```python
from build123d import *

# Parameters (mm, degrees)
SKETCH1_W           = 56
SKETCH1_H           = 37.25
BOSS_EXTRUDE1_DEPTH = 2
SKETCH2_W           = 56
SKETCH2_H           = 37.25
SKETCH2_W_2         = 52
SKETCH2_H_2         = 33.25
BOSS_EXTRUDE2_DEPTH = 8.5
SKETCH5_W           = 54
SKETCH5_H           = 35.25
SKETCH5_W_2         = 52
SKETCH5_H_2         = 33.25
CUT_EXTRUDE1_DEPTH  = 1
FILLET1_R           = 1
SKETCH7_W           = 30
SKETCH7_H           = 14
CUT_EXTRUDE3_DEPTH  = 10
SKETCH8_R           = 1.75
CUT_EXTRUDE4_DEPTH  = 10
SKETCH9_W           = 7
SKETCH9_H           = 6
CUT_EXTRUDE5_DEPTH  = 3
SKETCH10_W          = 10
SKETCH10_H          = 2.5
CUT_EXTRUDE6_DEPTH  = 3
FILLET2_R           = 0.5
FILLET3_R           = 1
FILLET5_R           = 0.2
CUT_EXTRUDE8_DEPTH  = 0.7
CUT_EXTRUDE10_DEPTH = 5
FILLET6_R           = 0.2


with BuildPart() as part:
    # Sketch1 → Boss-Extrude1 (new body)
    with BuildSketch(Plane(origin=(0, 0, 0), x_dir=(1, 0, 0), z_dir=(0, 1, 0))):
        with Locations((28, 18.625)):
            Rectangle(SKETCH1_W, SKETCH1_H)
    extrude(amount=BOSS_EXTRUDE1_DEPTH)

    # Sketch2 → Boss-Extrude2 (add)
    with BuildSketch(Plane(origin=(0, 2, 0), x_dir=(1, 0, 0), z_dir=(0, 1, 0))):
        with Locations((28, 18.625)):
            Rectangle(SKETCH2_W, SKETCH2_H)
        with Locations((28, 18.625)):
            Rectangle(SKETCH2_W_2, SKETCH2_H_2, mode=Mode.SUBTRACT)
    extrude(amount=BOSS_EXTRUDE2_DEPTH)

    # Sketch5 → Cut-Extrude1 (cut)
    with BuildSketch(Plane(origin=(0, 10.5, 0), x_dir=(1, 0, 0), z_dir=(0, 1, 0))):
        with Locations((28, 18.625)):
            Rectangle(SKETCH5_W, SKETCH5_H)
        with Locations((28, 18.625)):
            Rectangle(SKETCH5_W_2, SKETCH5_H_2, mode=Mode.SUBTRACT)
        with Locations((28, 18.625)):
            Rectangle(SKETCH5_W_2, SKETCH5_H_2)
    extrude(amount=-CUT_EXTRUDE1_DEPTH, mode=Mode.SUBTRACT)

    # Fillet1
    fillet1_edges = [part.edges().sort_by_distance(p)[0] for p in [
        (0, 5.25, -37.25),
        (56, 5.25, -37.25),
        (56, 5.25, 0),
        (0, 5.25, 0),
    ]]
    fillet(fillet1_edges, radius=FILLET1_R)

    # Sketch7 → Cut-Extrude3 (cut)
    with BuildSketch(Plane(origin=(0, 2, 0), x_dir=(1, 0, 0), z_dir=(0, 1, 0))):
        with Locations((31, 13)):
            Rectangle(SKETCH7_W, SKETCH7_H)
    extrude(amount=-CUT_EXTRUDE3_DEPTH, mode=Mode.SUBTRACT)

    # Sketch8 → Cut-Extrude4 (cut)
    with BuildSketch(Plane.XZ):
        with Locations((29.24999924, -23.74999914)):
            Circle(SKETCH8_R)
        with Locations((37.25000102, -23.74999914)):
            Circle(SKETCH8_R)
    extrude(amount=-CUT_EXTRUDE4_DEPTH, mode=Mode.SUBTRACT)

    # Sketch9 → Cut-Extrude5 (cut)
    with BuildSketch(Plane(origin=(0, 0, -37.25), x_dir=(-1, 0, 0), z_dir=(0, 0, -1))):
        with Locations((-47.5, 7.5)):
            Rectangle(SKETCH9_W, SKETCH9_H)
    extrude(amount=-CUT_EXTRUDE5_DEPTH, mode=Mode.SUBTRACT)

    # Sketch10 → Cut-Extrude6 (cut)
    with BuildSketch(Plane(origin=(0, 0, -37.25), x_dir=(-1, 0, 0), z_dir=(0, 0, -1))):
        with Locations((-39, 9.25)):
            Rectangle(SKETCH10_W, SKETCH10_H)
    extrude(amount=-CUT_EXTRUDE6_DEPTH, mode=Mode.SUBTRACT)

    # Fillet2
    fillet2_edges = [part.edges().sort_by_distance(p)[0] for p in [
        (16, 1, -6),
        (16, 1, -20),
        (46, 1, -20),
        (46, 1, -6),
    ]]
    fillet(fillet2_edges, radius=FILLET2_R)

    # Fillet3
    fillet3_edges = [part.edges().sort_by_distance(p)[0] for p in [
        (28, 0, -37.25),
        (0, 0, -18.625),
        (56, 0, -18.625),
        (28, 0, 0),
        (0.292893219, 0, -0.292893219),
        (0.292893219, 0, -36.957106781),
        (55.707106781, 0, -0.292893219),
        (55.707106781, 0, -36.957106781),
    ]]
    fillet(fillet3_edges, radius=FILLET3_R)

    # Fillet5
    fillet5_edges = [part.edges().sort_by_distance(p)[0] for p in [
        (51, 4.5, -36.25),
        (44, 4.5, -36.25),
        (44, 8, -36.25),
        (34, 8, -36.25),
    ]]
    fillet(fillet5_edges, radius=FILLET5_R)

    # Sketch12 → Cut-Extrude8 (cut)
    with BuildSketch(Plane(origin=(0, 9.5, 0), x_dir=(1, 0, 0), z_dir=(0, 1, 0))):
        Polygon((34, 35.25), (34, 36.25), (1, 36.25), (1, 1), (55, 1), (55, 36.25), (51, 36.25), (51, 35.25), (54, 35.25), (54, 2), (2, 2), (2, 35.25), align=None)
    extrude(amount=-CUT_EXTRUDE8_DEPTH, mode=Mode.SUBTRACT)

    # Sketch13 → Cut-Extrude10 (cut)
    with BuildSketch(Plane.ZY):
        Polygon((-18.625, 8.5), (-19.625, 8.5), (-19.625, 10.5), (-17.625, 10.5), (-17.625, 8.5), align=None)
    extrude(amount=-CUT_EXTRUDE10_DEPTH, mode=Mode.SUBTRACT)

    # Fillet6
    fillet6_edges = [part.edges().sort_by_distance(p)[0] for p in [
        (1, 8.5, -17.625),
        (1, 8.5, -19.625),
    ]]
    fillet(fillet6_edges, radius=FILLET6_R)


solid = part.part
```
Can you work these out from the model? Positions are in its coordinate system, mm. A direction names the side the tool comes from. Round coordinates to 2 decimals unless told otherwise and drop trailing zeros. Loops run counter-clockwise (first coordinate to the right, second up) from the corner with the lowest first, then second, coordinate; pieces in that order, holes last. Notation, with made-up numbers: M 49,70.5 L 107,70.5 A19 ccw 107,74.5 Z; hole C -34,13.5 d4. An arc over 180 degrees is marked long. Answer in a Markdown table with one row per item.
1. On a 3-axis mill with a long thin cutter (end or side, diameter ignored), from which of +Z, -Z, +X, -X, +Y, -Y can I reach the whole of each face in a straight line? I mean faces 5 (the face through (28, 5, -2)), 6 (the face through (0.5, 9.6, -17.625)), 7 (the face through (39, 8, -36)), 8 (the face through (46, 1, -13)). Say none if no direction works.
Established:
| item | result |
|---|---|
| face 5 | +Y |
| face 6 | -X, +Y |
| face 7 | -Z, +Y |
| face 8 | +Y, -Y |
2. If we section it at D-D, the plane z = -23.75: Please give me the cut outline in (x, y).
Established:
| item | result |
|---|---|
| outline | M 0,1 A1 ccw 1,0 L 27.5,0 L 27.5,2 L 2,2 L 2,8.8 L 1,8.8 L 1,10.5 L 0,10.5 Z; M 31,0 L 35.5,0 L 35.5,2 L 31,2 Z; M 39,0 L 55,0 A1 ccw 56,1 L 56,10.5 L 55,10.5 L 55,8.8 L 54,8.8 L 54,2 L 39,2 Z |
3. Please list where these lines run through material, in increasing order: line 1 (Z direction, x = 29.25, y = 1.3); line 2 (X direction, y = 10.25, z = -20.5); line 3 (Z direction, x = 6.5, y = 7.5). Write a range as from..to.
Established:
| item | result |
|---|---|
| line 1 | -37.25..-25.5, -22..-20, -6..0 |
| line 2 | 0..1, 55..56 |
| line 3 | -37.25..-35.25, -2..0 |
4. If we section it at B-B, the plane x = 29.25: Please give me the cut outline in (y, z).
Established:
| item | result |
|---|---|
| outline | M 0,-36.25 A1 ccw 1,-37.25 L 10.5,-37.25 L 10.5,-36.25 L 8.8,-36.25 L 8.8,-35.25 L 2,-35.25 L 2,-25.5 L 0,-25.5 Z; M 0,-22 L 2,-22 L 2,-20 L 0,-20 Z; M 0,-6 L 2,-6 L 2,-2 L 8.8,-2 L 8.8,-1 L 10.5,-1 L 10.5,0 L 1,0 A1 ccw 0,-1 Z |
5. I'm going to push flat-ended pins straight in: pin 1 Ø0.5 at (x, y) = (0.5, 9.5) entering from -Z; pin 2 Ø0.6 at (x, z) = (38.5, -36.5) entering from +Y; pin 3 Ø3 at (x, z) = (47, -26) entering from +Y; pin 4 Ø2 at (x, z) = (37.25, -23.75) entering from -Y. Where does each tip first touch, or does it pass through?
Established:
| item | result |
|---|---|
| pin 1 | z = -37.22 |
| pin 2 | y = 8 |
| pin 3 | y = 2 |
| pin 4 | through |
6. Thinking about a two-plate mould opening in X: for faces 1 (the face through (28, 6, -37.25)), 2 (the face through (56, 6, -18)), 3 (the face through (28, 10, -1)), 4 (the face through (31, 1, -20)), which applies, pulls with the +X half, pulls with the -X half, needs draft (parallel to the pull), parting line crosses it, or undercut?
Established:
| item | result |
|---|---|
| face 1 | needs draft |
| face 2 | pulls with the +X half |
| face 3 | undercut |
| face 4 | undercut |
7. If we section it at C-C, the plane x = 21.5: Please give me the cut outline in (y, z).
Established:
| item | result |
|---|---|
| outline | M 0,-36.25 A1 ccw 1,-37.25 L 10.5,-37.25 L 10.5,-36.25 L 8.8,-36.25 L 8.8,-35.25 L 2,-35.25 L 2,-20 L 0,-20 Z; M 0,-6 L 2,-6 L 2,-2 L 8.8,-2 L 8.8,-1 L 10.5,-1 L 10.5,0 L 1,0 A1 ccw 0,-1 Z |
8. If we section it at A-A, the plane z = -9.5: Please give me the cut outline in (x, y).
Established:
| item | result |
|---|---|
| outline | M 0,1 A1 ccw 1,0 L 16,0 L 16,2 L 2,2 L 2,8.8 L 1,8.8 L 1,10.5 L 0,10.5 Z; M 46,0 L 55,0 A1 ccw 56,1 L 56,10.5 L 55,10.5 L 55,8.8 L 54,8.8 L 54,2 L 46,2 Z |
